from build123d import *

# Parameters (mm, degrees)
F2_R = 100
F3_R = 5
F4_T = -2.5


with BuildPart() as f1:
    # F0 (on Top) → F1 (revolve)
    with BuildSketch(Plane.XY):
        Polygon((0, -300.5), (0, 0), (-13.75, 0), (-13.75, -63), (-37.6, -129), (-37.6, -300.5), align=None)
    revolve(axis=Axis((0, -150.25, 0), (0, -1, 0)))

    # F2
    f2_edges = [f1.edges().sort_by_distance(p)[0] for p in [
        (13.75, -63, 0),
        (37.6, -129, 0),
    ]]
    fillet(f2_edges, radius=F2_R)

    # F3
    f3_edges = [f1.edges().sort_by_distance(p)[0] for p in [
        (37.6, -300.5, 0),
    ]]
    fillet(f3_edges, radius=F3_R)

    # F4
    f4_openings = [f1.faces().sort_by_distance(p)[0] for p in [
        (0, 0, 0),
    ]]
    offset(amount=F4_T, openings=f4_openings)


solid = f1.part
CAD build for the part. Positions are in the model's coordinates, mm. A direction names the side the tool comes from. Give positions to 0.01 mm unless a question says otherwise; leave off trailing zeros. Order: outer loops, then holes, each group sorted by start corner. A loop starts at its lowest first (then second) coordinate and runs counter-clockwise, first axis right, second up. Notation, with made-up numbers: (62, 15.5) - (99, 15.5) arc R20 cw to (99, 42.5) - close; hole circle Ø9 at (6, 54). An arc over 180 degrees is marked (long way). Write each question's results on one line, items separated by ' | '.
1. Pull direction Y, two halves, no side cores. Call faces 1 (the face through (0, -300.5, 0)), 2 (the face through (8.151, -222.05, 36.706)), 3 (the face through (27.85, -222.05, 21.36)): released by +Y, released by -Y, zero draft, split by the parting line, or undercut.
Calculated:
face 1: released by -Y | face 2: zero draft | face 3: undercut
2. Pin check, flat tips, straight feed: pin 1 (6 mm diameter, centred on y = -247.5, z = 13.5, fed in from +X); pin 2 (8 mm diameter, centred on y = -249, z = 28, fed in from -X); pin 3 (1.5 mm diameter, centred on y = -260, z = -27.5, fed in from -X). Stop position of each tip, or through.
Calculated:
pin 1: stops at x = 36.1 | pin 2: stops at x = -28.94 | pin 3: stops at x = -26.42
3. Probe L1, parallel to X at y = -212, z = 0; L2, parallel to Z at x = 0, y = -29. List the from-to ranges inside material, lowest first. Write a range as from..to.
Calculated:
L1: x = -37.6..-35.1, 35.1..37.6 | L2: z = -13.75..-11.25, 11.25..13.75
4. 3-axis set-ups, long thin cutter, end or side, ignore diameter. For faces 4 (the face through (-11.3, 0, -2.1)), 5 (the face through (-19.17, -89.74, 7.95)), 6 (the face through (-6.34, -23.06, 12.2)): which of +Z, -Z, +X, -X, +Y, -Y reach the whole face in a straight line?
Calculated:
face 4: +Z, -Z, +X, -X, +Y | face 5: none | face 6: +Y
5. Saw through at A-A on y = -235. List the corners of the cut face in (x, z), and give its area (3 significant figures).
Calculated:
outline: circle Ø75.2 at (0, 0); hole circle Ø70.2 at (0, 0) | area: 571 mm2
